from build123d import *

# Parameters (mm, degrees)
SKETCH1_R           = 1.5
BOSS_EXTRUDE1_DEPTH = 3
FILLET1_R           = 5
FILLET2_R           = 5


with BuildPart() as part:
    # Sketch1 → Boss-Extrude1 (new body)
    with BuildSketch(Plane.XY):
        Polygon((6, 0), (-6, 0), (-6, 23.6), (-15, 23.6), (-15, 27.6), (15, 27.6), (15, 23.6), (6, 23.6), align=None)
        with Locations((0, 6.5)):
            Circle(SKETCH1_R, mode=Mode.SUBTRACT)
        with Locations((0, 21.5)):
            Circle(SKETCH1_R, mode=Mode.SUBTRACT)
    extrude(amount=BOSS_EXTRUDE1_DEPTH)

    # Fillet1
    fillet1_edges = [part.edges().sort_by_distance(p)[0] for p in [
        (-6, 23.6, 1.5),
    ]]
    fillet(fillet1_edges, radius=FILLET1_R)

    # Fillet2
    fillet2_edges = [part.edges().sort_by_distance(p)[0] for p in [
        (6, 23.6, 1.5),
    ]]
    fillet(fillet2_edges, radius=FILLET2_R)


solid = part.part
Source: CAD feature listing. Evaluate the final solid. Frame: model axes, mm. A direction names the side the tool comes from. Coordinates: 2 decimals unless noted, no trailing zeros. Order: outer loops, then holes, each group sorted by start corner. A loop starts at its lowest first (then second) coordinate and runs counter-clockwise, first axis right, second up.
Item 1: Pull-direction query (Y, two-part tool) for faces 1 (the face through (-13, 23.6, 1)), 2 (the face through (15, 26, 1)), 3 (the face through (0, 5, 1)); classes: pulls with the +Y half, pulls with the -Y half, needs draft (parallel to the pull), parting line crosses it, or undercut.
Output values:
face 1: pulls with the -Y half
face 2: needs draft
face 3: undercut
Item 2: Set-up query: faces 4 (the face through (13, 23.6, 1)), 5 (the face through (0, 0, 1)), 6 (the face through (-6, 9, 1)). Return all of +Z, -Z, +X, -X, +Y, -Y with unobstructed straight access to the full face (end or side cutting, diameter ignored); none if empty.
Output values:
face 4: +Z, -Z, +X, -Y
face 5: +Z, -Z, +X, -X, -Y
face 6: +Z, -Z, -X, -Y
Item 3: Cut plane B-B (y = 6.5). Return loops of the section in (x, z), plus the area to 3 significant figures.
Output values:
outline: (-6, 0) - (-1.5, 0) - (-1.5, 3) - (-6, 3) - close; (1.5, 0) - (6, 0) - (6, 3) - (1.5, 3) - close
area: 27.0 mm2
Item 4: Cut plane C-C (z = 0.65). Return loops of the section in (x, y).
Output values:
outline: (-15, 23.6) - (-11, 23.6) arc R5 cw to (-6, 18.6) - (-6, 0) - (6, 0) - (6, 18.6) arc R5 cw to (11, 23.6) - (15, 23.6) - (15, 27.6) - (-15, 27.6) - close; hole circle Ø3 at (0, 6.5); hole circle Ø3 at (0, 21.5)
Item 5: Cut plane A-A (x = 0). Return loops of the section in (y, z), plus the area to 3 significant figures.
Output values:
outline: (0, 0) - (5, 0) - (5, 3) - (0, 3) - close; (8, 0) - (20, 0) - (20, 3) - (8, 3) - close; (23, 0) - (27.6, 0) - (27.6, 3) - (23, 3) - close
area: 64.8 mm2
Item 6: First-contact query: P1, Ø2.5, axis at x = 0, y = 21.5, coming from the -Z side; P2, Ø0.9, axis at y = 8, z = 1.5, coming from the -X side. Flat tips, straight axial feed; report the tip coordinate or a pass-through.
Output values:
P1: passes through
P2: stops at x = -6
Item 7: Material intervals for line 1 (Y direction, x = 0, z = 1.05); line 2 (X direction, y = 13.75, z = 2.35); line 3 (Y direction, x = 11.25, z = 0.5), sorted ascending.
Output values:
line 1: y = 0 to 5, 8 to 20, 23 to 27.6
line 2: x = -6 to 6
line 3: y = 23.6 to 27.6
Item 8: Cut plane D-D (y = 18). Return loops of the section in (x, z), plus the area to 3 significant figures.
Output values:
outline: (-6, 0) - (6, 0) - (6, 3) - (-6, 3) - close
area: 36.0 mm2
